Read the model definition and answer for the solid it produces. Units are mm, in the model's axes. Face numbers are marked on the shaded views. A direction names the side the tool comes from. Coordinates: 2 decimals unless noted, no trailing zeros. Loops run counter-clockwise (first coordinate to the right, second up) from the corner with the lowest first, then second, coordinate; pieces in that order, holes last. Notation, with made-up numbers: (18.25, 41) -> (51.25, 41) arc R25 cw to (51.25, 73) -> close; hole circle Ø7 at (79, 51.25). An arc over 180 degrees is marked (long way). Answer as a JSON object with one key per item and string values. Group by question number.
1) Flat-ended cylindrical pins translate along their axes: P1, Ø12, axis at x = 29, z = 33, coming from the +Y side; P2, Ø4, axis at x = -3.5, z = 13.5, coming from the +Y side; P3, Ø19, axis at y = 34, z = 23, coming from the -X side. Find the tip coordinate at first contact, or state that the pin passes through.
2) Determine the mould class of the marked faces 1, 2 and 3 for opening direction Z: released by +Z, released by -Z, zero draft, split by the parting line, or undercut.
3) Section C-C, the plane y = 74 is taken. Give the vertices of the cut face in (x, z).
4) Which of the six approach directions +Z, -Z, +X, -X, +Y, -Y give full straight-line access (tool end or side, diameter ignored) to the marked faces 4, 5 and 6?
5) Consider probe 1 along Z at (x, y) = (3.5, 47); probe 2 along X at (y, z) = (70, 33.5); probe 3 along Y at (x, z) = (-5.5, 17). Determine where each line is inside the solid, lowest interval first. Write a range as [from, to].
6) Section D-D, the plane x = 16 is taken. Give the vertices of the cut face in (y, z), plus the area to 3 significant figures.
7) Section A-A, the plane z = 10 is taken. Give the vertices of the cut face in (x, y).
8) Section B-B, the plane z = 18 is taken. Give the vertices of the cut face in (x, y).
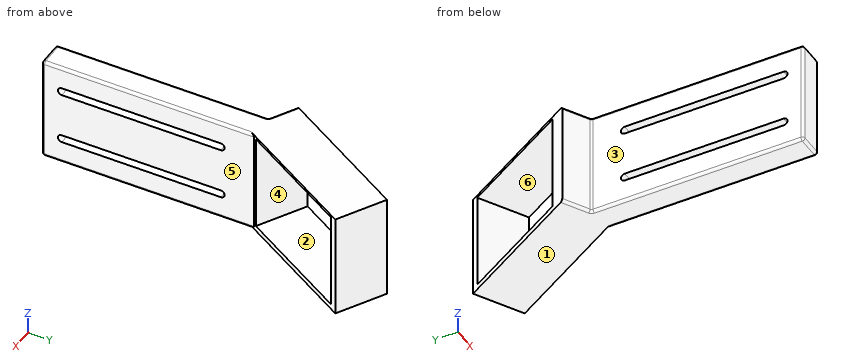
from build123d import *

# Parameters (mm, degrees)
BOSS_EXTRU_1_DEPTH      = 40
CONG_2_R                = 1
ENL_V_MAT_EXTRU_4_REACH = 147.362
ESQUISSE14_W            = 37
ESQUISSE14_H            = 48
ENL_V_MAT_EXTRU_5_DEPTH = 20


with BuildPart() as part:
    # Esquisse1 → Boss.-Extru.1 (new body)
    with BuildSketch(Plane.XY):
        Polygon((0, 0), (10, 0), (10, 80), (36, 125.033320997), (18.679491924, 135.033320997), (-9.820508076, 85.669872981), (0, 80), align=None)
    extrude(amount=BOSS_EXTRU_1_DEPTH)

    # Congé2
    cong_2_edges = [part.edges().sort_by_distance(p)[0] for p in [
        (0, 40, 0),
        (0, 80, 20),
        (10, 40, 40),
        (10, 0, 20),
        (0, 0, 20),
        (-4.910254038, 82.834936491, 40),
        (0, 40, 40),
        (-4.910254038, 82.834936491, 0),
        (5, 0, 40),
        (10, 40, 0),
        (5, 0, 0),
    ]]
    fillet(cong_2_edges, radius=CONG_2_R)

    # Esquisse13 → Enlèv. mat.-Extru.4 (cut, up to next)
    with BuildSketch(Plane.ZY, mode=Mode.PRIVATE) as enl_v_mat_extru_4_sk1:
        with BuildLine():
            Line((8.55, 7.5), (8.55, 67.5))
            ThreePointArc((8.55, 67.5), (10, 68.95), (11.45, 67.5))
            Line((11.45, 67.5), (11.45, 7.5))
            ThreePointArc((11.45, 7.5), (10, 6.05), (8.55, 7.5))
        make_face()
    enl_v_mat_extru_4_tool1 = extrude(enl_v_mat_extru_4_sk1.sketch, amount=-ENL_V_MAT_EXTRU_4_REACH, mode=Mode.PRIVATE) & part.part
    # Esquisse13 → Enlèv. mat.-Extru.4 (cut, up to next)
    with BuildSketch(Plane.ZY, mode=Mode.PRIVATE) as enl_v_mat_extru_4_sk2:
        with BuildLine():
            Line((28.55, 7.5), (28.55, 67.5))
            ThreePointArc((28.55, 67.5), (30, 68.95), (31.45, 67.5))
            Line((31.45, 67.5), (31.45, 7.5))
            ThreePointArc((31.45, 7.5), (30, 6.05), (28.55, 7.5))
        make_face()
    enl_v_mat_extru_4_tool2 = extrude(enl_v_mat_extru_4_sk2.sketch, amount=-ENL_V_MAT_EXTRU_4_REACH, mode=Mode.PRIVATE) & part.part
    add(enl_v_mat_extru_4_tool1.solids().sort_by_distance((0, 37.5, 10))[0], mode=Mode.SUBTRACT)
    add(enl_v_mat_extru_4_tool2.solids().sort_by_distance((0, 37.5, 30))[0], mode=Mode.SUBTRACT)

    # Esquisse14 → Enlèv. mat.-Extru.5 (cut)
    with BuildSketch(Plane(origin=(-44.461524227, 25.669872981, 0), x_dir=(0, 0, 1), z_dir=(-0.8660254037844419, 0.4999999999999945, 0))):
        with Locations((20.5, 99.55560496)):
            Rectangle(ESQUISSE14_W, ESQUISSE14_H)
    extrude(amount=-ENL_V_MAT_EXTRU_5_DEPTH, mode=Mode.SUBTRACT)


solid = part.part
Determined:
{
 "1": {"P1": "y = 132.54", "P2": "y = 90.42", "P3": "x = 0"},
 "2": {"face 1": "released by -Z", "face 2": "undercut", "face 3": "zero draft"},
 "3": {"outline": "(0, 1) arc R1 ccw to (1, 0) -> (9, 0) arc R1 ccw to (10, 1) -> (10, 39) arc R1 ccw to (9, 40) -> (1, 40) arc R1 ccw to (0, 39) -> close"},
 "4": {"face 4": "+X, +Y", "face 5": "+Z, -Z, +X, -Y", "face 6": "none"},
 "5": {"probe 1": "[0, 8.55], [11.45, 28.55], [31.45, 40]", "probe 2": "[0, 10]", "probe 3": "[83.18, 90.42]"},
 "6": {"outline": "(90.39, 0) -> (130.39, 0) -> (130.39, 2) -> (90.39, 2) -> close; (90.39, 39) -> (130.39, 39) -> (130.39, 40) -> (90.39, 40) -> close", "area": "120 mm²"},
 "7": {"outline": "(-9.82, 85.67) -> (-0.5, 80.29) arc R1 cw to (0, 79.42) -> (0, 68.95) -> (10, 68.95) -> (10, 80) -> (10.64, 81.1) -> (-6.68, 91.1) -> close; (0, 1) arc R1 ccw to (1, 0) -> (9, 0) arc R1 ccw to (10, 1) -> (10, 6.05) -> (0, 6.05) -> close; (17.32, 132.67) -> (34.64, 122.67) -> (36, 125.03) -> (18.68, 135.03) -> close"},
 "8": {"outline": "(-9.82, 85.67) -> (-0.5, 80.29) arc R1 cw to (0, 79.42) -> (0, 1) arc R1 ccw to (1, 0) -> (9, 0) arc R1 ccw to (10, 1) -> (10, 80) -> (10.64, 81.1) -> (-6.68, 91.1) -> close; (17.32, 132.67) -> (34.64, 122.67) -> (36, 125.03) -> (18.68, 135.03) -> close"}
}
